from build123d import *

# Parameters (mm, degrees)
SKETCH1_W           = 257.9
SKETCH1_H           = 165.1
SKETCH1_W_2         = 6.35
SKETCH1_H_2         = 7.62
BOSS_EXTRUDE1_DEPTH = 6
SKETCH2_R           = 1.778
CUT_EXTRUDE1_DEPTH  = 307.278337464
SKETCH3_W           = 42
SKETCH3_H           = 31.9913
SKETCH3_W_2         = 31.713
SKETCH3_H_2         = 64.0842
CUT_EXTRUDE2_DEPTH  = 307.278337464
FILLET1_R           = 5.08
FILLET2_R           = 2.54


with BuildPart() as part:
    # Sketch1 → Boss-Extrude1 (new body)
    with BuildSketch(Plane.XY):
        with Locations((128.95, 82.55)):
            Rectangle(SKETCH1_W, SKETCH1_H)
        with Locations((229.325, 157.8356)):
            Rectangle(SKETCH1_W_2, SKETCH1_H_2, mode=Mode.SUBTRACT)
        with Locations((61.05, 157.8356)):
            Rectangle(SKETCH1_W_2, SKETCH1_H_2, mode=Mode.SUBTRACT)
        with Locations((229.325, 71.3486)):
            Rectangle(SKETCH1_W_2, SKETCH1_H_2, mode=Mode.SUBTRACT)
        with Locations((61.05, 71.3486)):
            Rectangle(SKETCH1_W_2, SKETCH1_H_2, mode=Mode.SUBTRACT)
    extrude(amount=BOSS_EXTRUDE1_DEPTH)

    # Sketch2 → Cut-Extrude1 (cut, through all)
    with BuildSketch(Plane.XY.offset(6)):
        with Locations((245.2, 116.3447)):
            Circle(SKETCH2_R)
        with BuildLine():
            Line((4.23, 127.9712), (6.77, 127.9712))
            ThreePointArc((6.77, 127.9712), (8.3575, 126.3837), (6.77, 124.7962))
            Line((6.77, 124.7962), (4.23, 124.7962))
            ThreePointArc((4.23, 124.7962), (2.6425, 126.3837), (4.23, 127.9712))
        make_face()
        with BuildLine():
            Line((35.23, 127.9712), (37.77, 127.9712))
            ThreePointArc((37.77, 127.9712), (39.3575, 126.3837), (37.77, 124.7962))
            Line((37.77, 124.7962), (35.23, 124.7962))
            ThreePointArc((35.23, 124.7962), (33.6425, 126.3837), (35.23, 127.9712))
        make_face()
        with BuildLine():
            Line((35.23, 96.9712), (37.77, 96.9712))
            ThreePointArc((37.77, 96.9712), (39.3575, 95.3837), (37.77, 93.7962))
            Line((37.77, 93.7962), (35.23, 93.7962))
            ThreePointArc((35.23, 93.7962), (33.6425, 95.3837), (35.23, 96.9712))
        make_face()
        with BuildLine():
            Line((4.23, 96.9712), (6.77, 96.9712))
            ThreePointArc((6.77, 96.9712), (8.3575, 95.3837), (6.77, 93.7962))
            Line((6.77, 93.7962), (4.23, 93.7962))
            ThreePointArc((4.23, 93.7962), (2.6425, 95.3837), (4.23, 96.9712))
        make_face()
        with BuildLine():
            Line((19.73, 122.0087), (22.27, 122.0087))
            ThreePointArc((22.27, 122.0087), (33.395, 110.8837), (22.27, 99.7587))
            Line((22.27, 99.7587), (19.73, 99.7587))
            ThreePointArc((19.73, 99.7587), (8.605, 110.8837), (19.73, 122.0087))
        make_face()
    extrude(amount=-CUT_EXTRUDE1_DEPTH, mode=Mode.SUBTRACT)

    # Sketch3 → Cut-Extrude2 (cut, through all)
    with BuildSketch(Plane.XY.offset(6)):
        Polygon((61.087, 0), (61.087, 64.0842), (42, 64.0842), (42, 88.6587), (0, 88.6587), (0, 0), align=None)
        with Locations((21, 149.10435)):
            Rectangle(SKETCH3_W, SKETCH3_H)
        with Locations((242.0435, 32.0421)):
            Rectangle(SKETCH3_W_2, SKETCH3_H_2)
    extrude(amount=-CUT_EXTRUDE2_DEPTH, mode=Mode.SUBTRACT)

    # Fillet1
    fillet1_edges = [part.edges().sort_by_distance(p)[0] for p in [
        (61.087, 0, 3),
        (42, 88.6587, 3),
        (42, 64.0842, 3),
        (61.087, 64.0842, 3),
        (42, 165.1, 3),
        (42, 133.1087, 3),
        (226.187, 0, 3),
        (226.187, 64.0842, 3),
        (257.9, 64.0842, 3),
        (257.9, 165.1, 3),
    ]]
    fillet(fillet1_edges, radius=FILLET1_R)

    # Fillet2
    fillet2_edges = [part.edges().sort_by_distance(p)[0] for p in [
        (0, 88.6587, 3),
        (0, 133.1087, 3),
    ]]
    fillet(fillet2_edges, radius=FILLET2_R)


solid = part.part
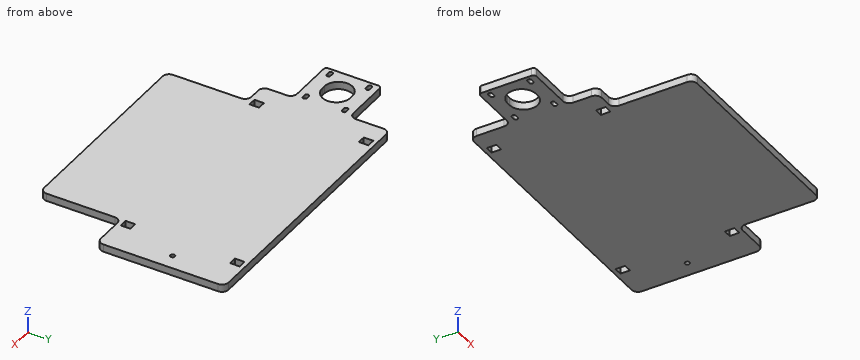
Geometry check sheet. Reference: the model listing, model coordinates, mm. Round coordinates to 2 decimals unless told otherwise and drop trailing zeros. Loops run counter-clockwise (first coordinate to the right, second up) from the corner with the lowest first, then second, coordinate; pieces in that order, holes last.
Item 1: Thickness scan on line 1 (X direction, y = 157, z = 2.2) (3 decimals); line 2 (Y direction, x = 58.5, z = 1.8); line 3 (Y direction, x = 245.2, z = 3). Record the ranges inside material, lowest first.
Item 2: Gauge pin test, flat ends, axial feed: pin 1 (1.8 mm diameter, centred on y = 159, z = 1.5, fed in from -X); pin 2 (1.3 mm diameter, centred on x = 20.5, z = 3, fed in from -Y); pin 3 (3 mm diameter, centred on x = 36.5, z = 4, fed in from +Y). Record the tip position at first contact, or that the pin passes through.
Item 3: Cross-section at C-C on z = 4. Count the separate pieces of the cut face and the enclosed holes in it, then the cut area to 3 significant figures.
Item 4: Cross-section at B-B on y = 31.5. Record the boundary of the cut face in (x, z).
Item 5: Cross-section at A-A on x = 239.5. Record the boundary of the cut face in (y, z), then the cut area to 3 significant figures.
Answer sheet:
1. line 1: x = 42 to 57.875, 64.225 to 226.15, 232.5 to 257.9
1. line 2: y = 63.43 to 67.54, 75.16 to 154.03, 161.65 to 165.1
1. line 3: y = 64.08 to 114.57, 118.12 to 165.1
2. pin 1: stops at x = 42
2. pin 2: stops at y = 88.66
2. pin 3: stops at y = 133.22
3. separate pieces: 1
3. enclosed holes: 10
3. area: 33,500 mm2
4. outline: (61.09, 0) - (226.19, 0) - (226.19, 6) - (61.09, 6) - close
5. outline: (64.08, 0) - (165.1, 0) - (165.1, 6) - (64.08, 6) - close
5. area: 606 mm2
